Verification items for the finished model (mm, model axes). Give positions to 0.01 mm unless a question says otherwise; leave off trailing zeros. Order: outer loops, then holes, each group sorted by start corner. A loop starts at its lowest first (then second) coordinate and runs counter-clockwise, first axis right, second up. Notation, with made-up numbers: (15.5, -14.5) -> (22.5, -14.5) arc R27 ccw to (22.5, 10.5) -> close; hole circle Ø8 at (9.25, -9). An arc over 180 degrees is marked (long way). Return JSON: item names as keys, results as strings. Group by question number.
(1) Cross-section at A-A on y = 15. Enter the section's corners in (x, z).
(2) Cross-section at B-B on x = 336. Enter the section's corners in (y, z).
(3) Thickness scan on line 1 along X through (y, z) = (15, 0.15); line 2 along Y through (x, z) = (430, 0.1); line 3 along Z through (x, y) = (678.5, 28). Record the ranges inside material, lowest first.
(4) Depth check by flat-ended pin: pin 1 Ø11.5 at (x, y) = (430, 15) entering from -Z; pin 2 Ø1 at (x, z) = (597.5, -7) entering from +Y; pin 3 Ø3 at (x, y) = (-92, 14) entering from +Z; pin 4 Ø13 at (x, y) = (129.5, 15.5) entering from -Z. Enter the tip coordinate at first touch or a pass-through.
from build123d import *

# Parameters (mm, degrees)
CUSTOM_TE_30X30X4_1_DEPTH    = 1800
ENL_V_MAT_EXTRU_4_DEPTH      = 1332.925298206
ENL_V_MAT_EXTRU_4_DEPTH_BACK = 1332.925298206
ESQUISSE15_R                 = 6.5


with BuildPart() as part:
    # Esquisse11 → Custom TE_30X30X4(1) (new body)
    with BuildSketch(Plane.ZY.offset(-900)):
        Polygon((-15, 0), (15, 0), (15, 4), (2, 4), (2, 30), (-2, 30), (-2, 4), (-15, 4), align=None)
    extrude(amount=CUSTOM_TE_30X30X4_1_DEPTH)

    # Esquisse15 → Enlèv. mat.-Extru.4 (cut, two sides: drawn at the far end of the back side and taken through both)
    with BuildSketch(Plane(origin=(430, 0, 50), x_dir=(1, 0, 0), z_dir=(0, 0, 1)).offset(-ENL_V_MAT_EXTRU_4_DEPTH_BACK)):
        with Locations(Location((0, 15, 0), (0, 0, 270))):
            Circle(ESQUISSE15_R)
    extrude(amount=ENL_V_MAT_EXTRU_4_DEPTH + ENL_V_MAT_EXTRU_4_DEPTH_BACK, mode=Mode.SUBTRACT)


solid = part.part
Verdict:
{
 "1": {"outline": "(-900, -2) -> (423.5, -2) -> (423.5, 2) -> (-900, 2) -> close; (436.5, -2) -> (900, -2) -> (900, 2) -> (436.5, 2) -> close"},
 "2": {"outline": "(0, -15) -> (4, -15) -> (4, -2) -> (30, -2) -> (30, 2) -> (4, 2) -> (4, 15) -> (0, 15) -> close"},
 "3": {"line 1": "-900 to 423.5, 436.5 to 900", "line 2": "0 to 8.5, 21.5 to 30", "line 3": "-2 to 2"},
 "4": {"pin 1": "through", "pin 2": "y = 4", "pin 3": "z = 2", "pin 4": "z = -2"}
}
